Part model, mm, in its own coordinate system. A direction names the side the tool comes from. Give positions to 0.01 mm unless a question says otherwise; leave off trailing zeros. Write each loop counter-clockwise with the first axis right and the second up, starting at its lowest first coordinate (ties: lowest second). Pieces come first, ordered by that corner, then holes. Notation, with made-up numbers: (57.5, 34) - (80.5, 34) arc R17 ccw to (80.5, 38) - close; hole circle Ø11 at (16, 88). An arc over 180 degrees is marked (long way). Answer in a Markdown table with one row per item. Add a question column.
1. Which spindle directions (+Z, -Z, +X, -X, +Y, -Y) get a long thin tool onto all of the face, cutting with end or side? Do faces 5 (the cylindrical face through (-2.1, -0.66, -5.85)), 6 (the conical face through (2.084, -3.589, 11.702)), 7 (the flat face through (0, 0, 11.089)). Say none if no direction does.
2. Drop flat-ended pins along their axis: pin 1 Ø1.5 at (x, z) = (1.5, 1) entering from +Y; pin 2 Ø3.5 at (x, y) = (0, 0) entering from +Z; pin 3 Ø1.5 at (x, z) = (-2.5, 5) entering from -Y. Give the stop position or say it passes through.
3. Band-saw the part on A-A on z = -2. Write the cut outline in (x, y), plus the area to 3 significant figures.
4. Pull direction Y, two halves, no side cores. Call faces 1 (the flat face through (0, 0, -36.711)), 2 (the conical face through (-2.07, -3.6, 11.7)), 3 (the conical face through (-2.084, 3.589, 11.702)), 4 (the cylindrical face through (-3, 0.1, 11.4)): released by +Y, released by -Y, zero draft, split by the parting line, or undercut.
5. Probe line 1 along Y through (x, z) = (0, 11.65); line 2 along Z through (x, y) = (3.25, 2); line 3 along Z through (x, y) = (-1, 0.25). List the from-to ranges inside material, lowest first.
Autodesk Inventor part; units mm, degrees
ref_plane "MSC_PF1" through (0, 0, 0) normal (0, 1, 0) x (-1, 0, 0)
ref_plane "MSC_PT1" through (0, 0, 8.2892) normal (0, 0, -1) x (-1, 0, 0)
ref_plane "YZ Plane" through (0, 0, 0) normal (1, 0, 0) x (0, 1, 0)
sketch "Sketch2" plane through (0, 0, 0) normal (0, 1, 0) x (-1, 0, 0)
  line L0 (0, 8.2892) -> (0, -36.7108)
  line L1 (0, -36.7108) -> (2.1, -36.7108)
  line L2 (2.5, -36.3108) -> (2.5, -20.7108)
  line L3 (2.5, -20.7108) -> (2.2, -20.1912)
  line L4 (2.2, -20.1912) -> (2.2, 8.2892)
  line L5 (2.2, 8.2892) -> (0, 8.2892)
  line L6 (2.1, -36.7108) -> (2.5, -36.3108)
  line L7 (2.5, -36.7108) -> (2.5, -37.2765)
  line L8 (0, -46.3897) -> (0, 17.4023)
  dimension "Ds" = 4.4
  dimension "NND" = 5
  dimension "b" = 16
  dimension "d3" = 30
  dimension "d5" = 45
  dimension "PTC" = 0.8
  dimension "NLG" = 45
revolve "Revolution1" add sketch "Sketch2" angle 360 about axis through (0, 0, 8.2892) along (0, 0, -1)
sketch "Sketch3" plane through (0, 0, 8.2892) normal (0, 0, 1) x (1, 0, 0)
  circle A0 centre (0, 0) radius 2.2
  line L0 (0, 4) -> (2.3094, 4)
  line L1 (2.3094, 4) -> (4.6188, 0)
  line L2 (4.6188, 0) -> (0, 0)
  line L3 (0, 0) -> (0, 4)
  line L4 (0, 4) -> (-2.3094, 4)
  line L5 (-2.3094, 4) -> (-4.6188, 0)
  line L6 (0, -4) -> (2.3094, -4)
  line L7 (2.3094, -4) -> (4.6188, 0)
  line L8 (-2.3094, -4) -> (-4.6188, 0)
  line L9 (0, -4) -> (-2.3094, -4)
  dimension "d9" = 60
  dimension "ParS" = 8
  dimension "msp_d11" = 8
extrude "Extrusion1" add sketch "Sketch3" along normal blind 3.5
sketch "Sketch4" plane through (0, 0, 0) normal (0, 1, 0) x (-1, 0, 0)
  line L0 (-4, 11.7892) -> (-4.6188, 11.7892)
  line L1 (-4.6188, 11.7892) -> (-4.6188, 11.4319)
  line L2 (-4.6188, 11.4319) -> (-4, 11.7892)
  line L3 (0, 4.4398) -> (0, 31.3854)
  line L4 (0, 27.536) -> (0, 27.1787)
  line L5 (-4.6188, 8.2892) -> (-4.6188, 11.7892)
  line L6 (-2.3094, 11.7892) -> (-4.6188, 11.7892)
  dimension "d14" = 30
  dimension "msp_d15" = 8
revolve "Revolution2" cut sketch "Sketch4" angle 360 about axis through (0, 0, 27.536) along (0, 0, -1)
sketch "Sketch5" plane through (0, 0, 11.7892) normal (0, 0, 1) x (1, 0, 0)
  arc A0 (3.4641, 2) -> (0, 4) centre (0, 0) ccw
  circle A1 centre (0, 0) radius 3
  dimension "d27" = 6
extrude "Extrusion2" cut sketch "Sketch5" against normal blind 0.7
thread "Thread1"
ref_plane "MSC_PF1" through (0, 0, 0) normal (0, 1, 0) x (-1, 0, 0)
ref_plane "MSC_PT1" through (0, 0, 8.2892) normal (0, 0, -1) x (-1, 0, 0)
fillet "Fillet1" radius 0.2 1 edges at (2.2, 0, 8.2892)
equation "\"msp_d11\" = ParS"
equation "\"msp_d15\" = ParS"
equation "\"d27\" = 0.75 * ParS"
equation "\"d28\" = 0.2 * ParK"
equation "\"d30\" = r"
equation "\"msp_d17\" = b"
equation "\"r\" = 0.2"
equation "\"THREADDIA\" = NND"
properties part number "ISO 4015 - M5 x 45" material "Stainless Steel, 440C"
Values:
| question | item | result |
|---|---|---|
| 1 | face 5 | none |
| 1 | face 6 | +Z, +X, -Y |
| 1 | face 7 | +Z |
| 2 | pin 1 | stops at y = 2.07 |
| 2 | pin 2 | stops at z = 11.09 |
| 2 | pin 3 | stops at y = -1.33 |
| 3 | outline | circle Ø4.4 at (0, 0) |
| 3 | area | 15.2 mm² |
| 4 | face 1 | zero draft |
| 4 | face 2 | released by -Y |
| 4 | face 3 | released by +Y |
| 4 | face 4 | undercut |
| 5 | line 1 | y = -4 to -3, 3 to 4 |
| 5 | line 2 | z = 8.29 to 11.79 |
| 5 | line 3 | z = -36.71 to 11.09 |
